```python
from build123d import *

# Parameters (mm, degrees)
SKETCH1_W           = 69.85
SKETCH1_H           = 57.15
BOSS_EXTRUDE1_DEPTH = 3.175
SKETCH2_R           = 4.776740808
SKETCH2_R_2         = 4.7625
BOSS_EXTRUDE2_DEPTH = 3.175
SKETCH3_R           = 2.4892
CUT_EXTRUDE1_DEPTH  = 54.678109207
SKETCH4_R           = 3.175
SKETCH4_R_2         = 4.7625
CUT_EXTRUDE2_DEPTH  = 54.678109207
SKETCH5_R           = 6.35
SKETCH5_R_2         = 7.9375
BOSS_EXTRUDE3_DEPTH = 3.175
SKETCH6_R           = 4.7625
SKETCH6_R_2         = 3.175
CUT_EXTRUDE3_DEPTH  = 54.959070443


with BuildPart() as part:
    # Sketch1 → Boss-Extrude1 (new body)
    with BuildSketch(Plane.XY):
        Rectangle(SKETCH1_W, SKETCH1_H)
    extrude(amount=BOSS_EXTRUDE1_DEPTH)

    # Sketch2 → Boss-Extrude2 (add)
    with BuildSketch(Plane.XY.offset(3.175)):
        with Locations((-36.080944449, 29.359475258)):
            Circle(SKETCH2_R)
        with Locations((35.832665303, 29.636957013)):
            Circle(SKETCH2_R_2)
        with Locations((35.864779118, -29.608646076)):
            Circle(SKETCH2_R_2)
        with Locations((-36.322, -29.590559194)):
            Circle(SKETCH2_R_2)
    extrude(amount=-BOSS_EXTRUDE2_DEPTH)

    # Sketch3 → Cut-Extrude1 (cut, through all)
    with BuildSketch(Plane.XY.offset(3.175)):
        with Locations((-36.080944449, 29.359475258)):
            Circle(SKETCH3_R)
        with Locations((35.832665303, 29.636957013)):
            Circle(SKETCH3_R)
        with Locations((35.864779118, -29.608646076)):
            Circle(SKETCH3_R)
        with Locations((-36.322, -29.590559194)):
            Circle(SKETCH3_R)
    extrude(amount=-CUT_EXTRUDE1_DEPTH, mode=Mode.SUBTRACT)

    # Sketch4 → Cut-Extrude2 (cut, through all)
    with BuildSketch(Plane.XY.offset(3.175)):
        with Locations((-8.73125, -0.039106259)):
            Circle(SKETCH4_R)
        with Locations((8.73125, 0.002745202)):
            Circle(SKETCH4_R_2)
    extrude(amount=-CUT_EXTRUDE2_DEPTH, mode=Mode.SUBTRACT)

    # Sketch5 → Boss-Extrude3 (add)
    with BuildSketch(Plane.XY.offset(3.175)):
        with Locations((-8.73125, -0.039106259)):
            Circle(SKETCH5_R)
        with Locations((8.73125, 0.002745202)):
            Circle(SKETCH5_R_2)
    extrude(amount=BOSS_EXTRUDE3_DEPTH)

    # Sketch6 → Cut-Extrude3 (cut, through all)
    with BuildSketch(Plane.XY.offset(6.35)):
        with Locations((8.73125, 0.002745202)):
            Circle(SKETCH6_R)
        with Locations((-8.73125, -0.039106259)):
            Circle(SKETCH6_R_2)
    extrude(amount=-CUT_EXTRUDE3_DEPTH, mode=Mode.SUBTRACT)


solid = part.part
```
CAD build for the part. Positions are in the model's coordinates, mm. A direction names the side the tool comes from. Round coordinates to 2 decimals unless told otherwise and drop trailing zeros. Order: outer loops, then holes, each group sorted by start corner. A loop starts at its lowest first (then second) coordinate and runs counter-clockwise, first axis right, second up.
Q1. Drop flat-ended pins along their axis: pin 1 (1.5 mm diameter, centred on x = -33, z = 2.5, fed in from -Y); pin 2 (4 mm diameter, centred on x = 14, y = 20, fed in from +Z) (3 decimals); pin 3 (2.5 mm diameter, centred on x = -4.5, z = 1.5, fed in from +Y) (3 decimals); pin 4 (4 mm diameter, centred on x = 32, y = -6, fed in from -Z). Give the stop position or say it passes through.
Q2. Slice it at C-C (z = 5). State how many separate pieces and enclosed holes the cut face has, and give its area (3 significant figures).
Q3. Slice it at A-A (y = -1). Write the cut outline in (x, z) (3 decimals).
Q4. Which spindle directions (+Z, -Z, +X, -X, +Y, -Y) get a long thin tool onto all of the face, cutting with end or side? Do faces 1 (the cylindrical face through (16.3, 2.4, 4.7)), 2 (the cylindrical face through (-38.81, -29.48, 1.61)). Say none if no direction does.
Q5. Wall check: L1, parallel to Y at x = -9, z = 4.5; L2, parallel to Y at x = -9, z = 0.5 (1 decimal); L3, parallel to Y at x = 28.5, z = 2 (3 decimals). Give the ranges that are in metal, low to high.
Q6. Slice it at D-D (x = -29). Write the cut outline in (y, z) (3 decimals), and give its area (3 significant figures).
Q7. Slice it at B-B (x = -8). Write the cut outline in (y, z) (3 decimals).
Q8. Two-plate mould, pull along Y, no slides. Class faces 3 (the cylindrical face through (-13.77, -3.903, 4.74)), 4 (the cylindrical face through (-37.916, 31.042, 1.61)), 5 (the flat face through (-12, -1, 6.35)): pulls with the +Y half, pulls with the -Y half, needs draft (parallel to the pull), parting line crosses it, or undercut.
Results below:
1. pin 1: stops at y = -33.6
1. pin 2: stops at z = 3.175
1. pin 3: stops at y = 28.575
1. pin 4: stops at z = 0
2. separate pieces: 2
2. enclosed holes: 2
2. area: 222 mm2
3. outline: (-34.925, 0) - (-11.757, 0) - (-11.757, 6.35) - (-15.008, 6.35) - (-15.008, 3.175) - (-34.925, 3.175) - close; (-5.705, 0) - (4.076, 0) - (4.076, 6.35) - (0.857, 6.35) - (0.857, 3.175) - (-2.454, 3.175) - (-2.454, 6.35) - (-5.705, 6.35) - close; (13.387, 0) - (34.925, 0) - (34.925, 3.175) - (16.605, 3.175) - (16.605, 6.35) - (13.387, 6.35) - close
4. face 1: +Z
4. face 2: +Z, -Z
5. L1: y = -6.38 to -3.2, 3.12 to 6.31
5. L2: y = -28.6 to -3.2, 3.1 to 28.6
5. L3: y = -28.575 to 28.575
6. outline: (-28.575, 0) - (28.575, 0) - (28.575, 3.175) - (-28.575, 3.175) - close
6. area: 181 mm2
7. outline: (-28.575, 0) - (-3.129, 0) - (-3.129, 6.35) - (-6.347, 6.35) - (-6.347, 3.175) - (-28.575, 3.175) - close; (3.051, 0) - (28.575, 0) - (28.575, 3.175) - (6.269, 3.175) - (6.269, 6.35) - (3.051, 6.35) - close
8. face 3: parting line crosses it
8. face 4: undercut
8. face 5: needs draft
